Geometry check sheet. Reference: the model listing, model coordinates, mm. A direction names the side the tool comes from. Give positions to 0.01 mm unless a question says otherwise; leave off trailing zeros. Loops run counter-clockwise (first coordinate to the right, second up) from the corner with the lowest first, then second, coordinate; pieces in that order, holes last. Notation, with made-up numbers: (41.25, 51.5) -> (61.25, 51.5) arc R20 ccw to (61.25, 78.5) -> close; hole circle Ø3 at (-33.75, 55). An arc over 180 degrees is marked (long way). One line per item, written item: value. Start each with the question number.
(1) Sectioned sample at B-B, the plane y = 53.5. Record the cut outline in (x, z), then the cut area to 3 significant figures.
(2) Gauge pin test, flat ends, axial feed: pin 1 Ø0.9 at (x, z) = (7.5, 1.5) entering from +Y; pin 2 Ø10.5 at (y, z) = (-27.5, -26) entering from -X; pin 3 Ø7 at (x, y) = (5, -21) entering from -Z. Record the tip position at first contact, or that the pin passes through.
(3) Scan lines: line 1 along Y through (x, z) = (13, 0.9); line 2 along Y through (x, z) = (35.5, -32); line 3 along Z through (x, y) = (53, 15). Record each from-to range of solid material in increasing order. Write a range as from..to.
(4) Sectioned sample at A-A, the plane x = -15. Record the cut outline in (y, z).
(5) Sectioned sample at C-C, the plane y = -14.5. Record the cut outline in (x, z).
(6) Sectioned sample at D-D, the plane y = 6.5. Record the cut outline in (x, z), then the cut area to 3 significant figures.
(7) Tool access check on faces 5 (the face through (-6, 23, 0)), 6 (the face through (40, 58, -18)), 7 (the face through (63.387, 70.244, -11.458)), 8 (the face through (34, -39.5, -18)). Record the directions out of +Z, -Z, +X, -X, +Y, -Y that give a thin tool (end or side, any length) a straight path to the whole face; none if there is none.
(8) Draft check along Y on faces 1 (the face through (44.5, 1.31, -25.85)), 2 (the face through (-6, -23, 0)), 3 (the face through (2, -18.5, -15)), 4 (the face through (2, 18.5, -15)). Enter one of: pulls with the +Y half, pulls with the -Y half, needs draft (parallel to the pull), parting line crosses it, or undercut.
from build123d import *

# Parameters (mm, degrees)
SKETCH_1_W          = 80
SKETCH_1_H          = 55
EXTRUDE_1_DEPTH     = 3
SKETCH_2_R          = 1.55
CUT_EXTRUDE_1_DEPTH = 24.5
SKETCH_3_W          = 3
SKETCH_3_H          = 55
EXTRUDE_2_DEPTH     = 1.5
SKETCH_5_W          = 3
SKETCH_5_H          = 55
EXTRUDE_3_DEPTH     = 50
SKETCH_6_W          = 51.5
SKETCH_6_H          = 3
EXTRUDE_4_DEPTH     = 50
SKETCH_7_W          = 51.5
SKETCH_7_H          = 3
EXTRUDE_5_DEPTH     = 50
SKETCH_8_W          = 51.5
SKETCH_8_H          = 155
EXTRUDE_6_DEPTH     = 40
EXTRUDE_7_DEPTH     = 12
CUT_EXTRUDE_2_DEPTH = 184
SKETCH_13_R         = 90
CUT_EXTRUDE_3_DEPTH = 92
SKETCH_14_W         = 68
SKETCH_14_H         = 37
EXTRUDE_8_DEPTH     = 40
CUT_EXTRUDE_4_DEPTH = 56


with BuildPart() as part:
    # Sketch 1 → Extrude 1 (new body)
    with BuildSketch(Plane.XY):
        Rectangle(SKETCH_1_W, SKETCH_1_H)
    extrude(amount=EXTRUDE_1_DEPTH)

    # Sketch 2 → Cut-Extrude 1 (cut)
    with BuildSketch(Plane(origin=(0, 0, 0), x_dir=(-1, 0, 0), z_dir=(0, 0, -1))):
        with Locations((37, 25)):
            Circle(SKETCH_2_R)
        with Locations((37, -25)):
            Circle(SKETCH_2_R)
        with Locations((-13, 25)):
            Circle(SKETCH_2_R)
        with Locations((-13, -25)):
            Circle(SKETCH_2_R)
    extrude(amount=-CUT_EXTRUDE_1_DEPTH, mode=Mode.SUBTRACT)



with BuildPart() as body_2:
    # Sketch 3 → Extrude 2 (new body)
    with BuildSketch(Plane(origin=(40, 0, 0), x_dir=(0, 0, -1), z_dir=(1, 0, 0))):
        with Locations((-1.5, 0)):
            Rectangle(SKETCH_3_W, SKETCH_3_H)
    extrude(amount=EXTRUDE_2_DEPTH)

    # Sketch 5 → Extrude 3 (add)
    with BuildSketch(Plane(origin=(41.5, 0, 0), x_dir=(0, 0, -1), z_dir=(1, 0, 0))):
        with Locations((-1.5, 0)):
            Rectangle(SKETCH_5_W, SKETCH_5_H)
    extrude(amount=EXTRUDE_3_DEPTH)


with BuildPart() as part_1:
    add(part.part)

    add(body_2.part)  # Extrude 4 merges body 2
    # Sketch 6 → Extrude 4 (add)
    with BuildSketch(Plane(origin=(0, 27.5, 0), x_dir=(1, 0, 0), z_dir=(0, 1, 0))):
        with Locations((65.75, -1.5)):
            Rectangle(SKETCH_6_W, SKETCH_6_H)
    extrude(amount=EXTRUDE_4_DEPTH)

    # Sketch 7 → Extrude 5 (add)
    with BuildSketch(Plane.XZ.offset(27.5)):
        with Locations((65.75, 1.5)):
            Rectangle(SKETCH_7_W, SKETCH_7_H)
    extrude(amount=EXTRUDE_5_DEPTH)

    # Sketch 8 → Extrude 6 (add)
    with BuildSketch(Plane(origin=(0, 0, 0), x_dir=(-1, 0, 0), z_dir=(0, 0, -1))):
        with Locations((-65.75, 0)):
            Rectangle(SKETCH_8_W, SKETCH_8_H)
    extrude(amount=EXTRUDE_6_DEPTH)

    # Sketch 9 → Extrude 7 (add)
    with BuildSketch(Plane.ZY.offset(-40)):
        Polygon((-40, 39.5), (3, 39.5), (3, 27.5), (0, 27.5), (0, -27.5), (3, -27.5), (3, -39.5), (-40, -39.5), align=None)
    extrude(amount=EXTRUDE_7_DEPTH)

    # Sketch 10 → Cut-Extrude 2 (cut)
    with BuildSketch(Plane(origin=(0, 77.5, 0), x_dir=(1, 0, 0), z_dir=(0, 1, 0))):
        Polygon((56.5, 15), (91.5, -3), (47.242857143, -3), align=None)
    extrude(amount=-CUT_EXTRUDE_2_DEPTH, mode=Mode.SUBTRACT)

    # Sketch 13 → Cut-Extrude 3 (cut, symmetric)
    with BuildSketch(Plane(origin=(17.918657198, 0, -34.841833441), x_dir=(0.889287802, 0, 0.457348013), z_dir=(-0.457348013, 0, 0.889287802))):
        with Locations((117.74187795, 0)):
            Circle(SKETCH_13_R)
    extrude(amount=CUT_EXTRUDE_3_DEPTH, both=True, mode=Mode.SUBTRACT)

    # Sketch 14 → Extrude 8 (add)
    with BuildSketch(Plane(origin=(0, 0, 0), x_dir=(-1, 0, 0), z_dir=(0, 0, -1))):
        with Locations((6, 0)):
            Rectangle(SKETCH_14_W, SKETCH_14_H)
    extrude(amount=EXTRUDE_8_DEPTH)

    # Sketch 16 → Cut-Extrude 4 (cut)
    with BuildSketch(Plane(origin=(0, 18.5, 0), x_dir=(1, 0, 0), z_dir=(0, 1, 0))):
        Polygon((-40, 5.848570226), (19.210183994, 40), (-40, 40), align=None)
    extrude(amount=-CUT_EXTRUDE_4_DEPTH, mode=Mode.SUBTRACT)


solid = part_1.part
Calculated:
1. outline: (40, -40) -> (71.59, -40) -> (58.27, -14.09) -> (56.5, -15) -> (47.24, 3) -> (40, 3) -> close
1. area: 844 mm2
2. pin 1: stops at y = 27.5
2. pin 2: stops at x = 28
2. pin 3: stops at z = -33.22
3. line 1: y = -27.5..-26.55, -23.45..23.45, 26.55..27.5
3. line 2: y = -39.5..39.5
3. line 3: z = -40..-39.65
4. outline: (-27.5, 0) -> (-18.5, 0) -> (-18.5, -20.27) -> (18.5, -20.27) -> (18.5, 0) -> (27.5, 0) -> (27.5, 3) -> (-27.5, 3) -> close
5. outline: (-40, -5.85) -> (19.21, -40) -> (53.09, -40) -> (30.97, 3) -> (-40, 3) -> close
6. outline: (-40, -5.85) -> (19.21, -40) -> (52.03, -40) -> (29.92, 3) -> (-40, 3) -> close
6. area: 2,470 mm2
7. face 5: -Z, -X, +Y
7. face 6: +Z, -Z, -X, +Y
7. face 7: +Z, +Y, -Y
7. face 8: +Z, -Z, -X, -Y
8. face 1: undercut
8. face 2: needs draft
8. face 3: pulls with the -Y half
8. face 4: pulls with the +Y half
